Input: part model. Units: mm. Frame: model coordinates. Face numbers are marked on the shaded views. A direction names the side the tool comes from. Coordinates: 2 decimals unless noted, no trailing zeros. Write each loop counter-clockwise with the first axis right and the second up, starting at its lowest first coordinate (ties: lowest second). Pieces come first, ordered by that corner, then holes.
1) Section query D-D (z = -21). Output: boundary loops of the cut face in (x, y).
2) Section query C-C (x = -17.5). Output: boundary loops of the cut face in (y, z).
3) Set-up query: the marked faces 5, 6, 7, 8 and 9. Return all of +Z, -Z, +X, -X, +Y, -Y with unobstructed straight access to the full face (end or side cutting, diameter ignored); none if empty.
4) Pin query (flat end, axial travel): pin 1 Ø2 at (y, z) = (15.5, -19.5) entering from -X; pin 2 Ø8 at (x, y) = (19, 10) entering from -Z; pin 3 Ø4 at (y, z) = (8.5, -29.5) entering from +X. Return the tip coordinate at first contact, or that it passes through.
5) Draft query along Z for the marked faces 1, 2, 3 and 4. Return one class per face: pulls with the +Z half, pulls with the -Z half, needs draft (parallel to the pull), parting line crosses it, or undercut.
6) Line query: L1, parallel to X at y = 4.25, z = -55.5; L2, parallel to Y at x = 63.5, z = -45; L3, parallel to Z at x = 10, y = 3.25. Output: solid intervals per line, ascending.
7) Section query A-A (y = 8.5). Output: boundary loops of the cut face in (x, z).
8) Section query B-B (z = -47). Output: boundary loops of the cut face in (x, y), then the cut area to 3 significant figures.
from build123d import *

# Parameters (mm, degrees)
DODANIE_WYCI_GNI_CIE1_DEPTH = 16.6
SZKIC2_W                    = 102
SZKIC2_H                    = 66
DODANIE_WYCI_GNI_CIE3_DEPTH = 2.5
SZKIC4_W                    = 19.615634033
SZKIC4_H                    = 31.453270058
WYTNIJ_WYCI_GNI_CIE2_DEPTH  = 12.5


with BuildPart() as part:
    # Szkic1 → Dodanie-wyciągnięcie1 (new body)
    with BuildSketch(Plane(origin=(0, 0, 0), x_dir=(1, 0, 0), z_dir=(0, 1, 0))):
        with BuildLine():
            Line((-29.315960912, -4.201954397), (52.684039088, -4.201954397))
            Line((52.684039088, -4.201954397), (52.684039088, 12.548045603))
            ThreePointArc((52.684039088, 12.548045603), (65.934039088, 25.798045603), (52.684039088, 39.048045603))
            Line((52.684039088, 39.048045603), (52.684039088, 55.798045603))
            Line((52.684039088, 55.798045603), (-29.315960912, 55.798045603))
            Line((-29.315960912, 55.798045603), (-29.315960912, -4.201954397))
        make_face()
    extrude(amount=DODANIE_WYCI_GNI_CIE1_DEPTH)

    # Szkic2 → Dodanie-wyciągnięcie3 (add)
    with BuildSketch(Plane(origin=(0, 16.6, 0), x_dir=(1, 0, 0), z_dir=(0, 1, 0))):
        with Locations((18.184039088, 25.798045603)):
            Rectangle(SZKIC2_W, SZKIC2_H)
    extrude(amount=DODANIE_WYCI_GNI_CIE3_DEPTH)

    # Szkic4 → Wytnij-wyciągnięcie2 (cut)
    with BuildSketch(Plane.XZ):
        with Locations((-11.960019209, -27.124412261)):
            Rectangle(SZKIC4_W, SZKIC4_H)
    extrude(amount=-WYTNIJ_WYCI_GNI_CIE2_DEPTH, mode=Mode.SUBTRACT)


solid = part.part
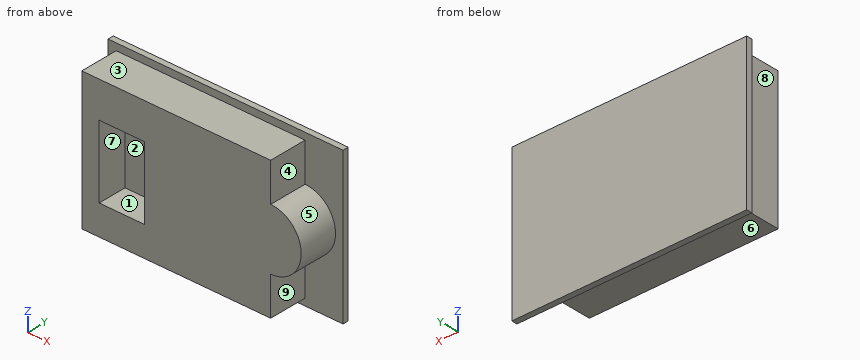
Answer:
1. outline: (-32.82, 16.6) - (-29.32, 16.6) - (-29.32, 0) - (-21.77, 0) - (-21.77, 12.5) - (-2.15, 12.5) - (-2.15, 0) - (65.03, 0) - (65.03, 16.6) - (69.18, 16.6) - (69.18, 19.1) - (-32.82, 19.1) - close
2. outline: (0, -55.8) - (16.6, -55.8) - (16.6, -58.8) - (19.1, -58.8) - (19.1, 7.2) - (16.6, 7.2) - (16.6, 4.2) - (0, 4.2) - (0, -11.4) - (12.5, -11.4) - (12.5, -42.85) - (0, -42.85) - close
3. face 5: +X, -Y
3. face 6: -Z, +X, -X, -Y
3. face 7: -Y
3. face 8: +Z, -Z, -X, -Y
3. face 9: -Z, +X, -Y
4. pin 1: stops at x = -29.32
4. pin 2: stops at z = -55.8
4. pin 3: stops at x = 65.82
5. face 1: undercut
5. face 2: undercut
5. face 3: pulls with the +Z half
5. face 4: needs draft
6. L1: x = -29.32 to 52.68
6. L2: y = 16.6 to 19.1
6. L3: z = -55.8 to 4.2
7. outline: (-29.32, -55.8) - (52.68, -55.8) - (52.68, -39.05) arc R13.25 ccw to (52.68, -12.55) - (52.68, 4.2) - (-29.32, 4.2) - close; hole (-21.77, -42.85) - (-2.15, -42.85) - (-2.15, -11.4) - (-21.77, -11.4) - close
8. outline: (-32.82, 16.6) - (-29.32, 16.6) - (-29.32, 0) - (52.68, 0) - (52.68, 16.6) - (69.18, 16.6) - (69.18, 19.1) - (-32.82, 19.1) - close
8. area: 1,620 mm2
